Geometry check sheet. Reference: the model listing, model coordinates, mm. Face numbers are marked on the shaded views. A direction names the side the tool comes from. Coordinates: 2 decimals unless noted, no trailing zeros. Write each loop counter-clockwise with the first axis right and the second up, starting at its lowest first coordinate (ties: lowest second). Pieces come first, ordered by that corner, then holes. Notation, with made-up numbers: (-36.75, 60.5) -> (-30.75, 60.5) arc R29 cw to (-30.75, 89.5) -> close; hole circle Ø5 at (82, -12). An arc over 180 degrees is marked (long way). Answer as CSV lines item,"result".
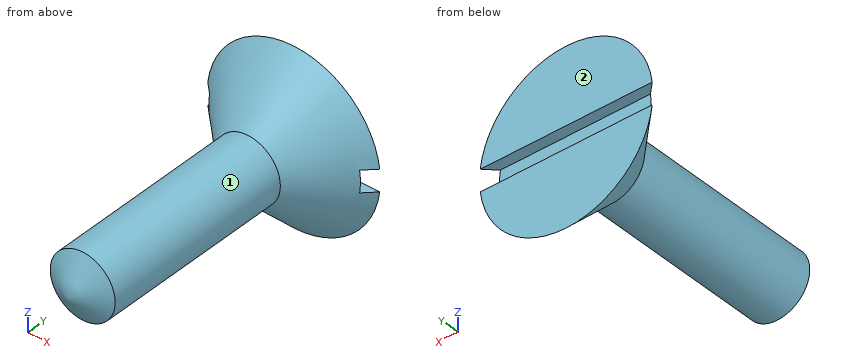
```python
from build123d import *

# Parameters (mm, degrees)
CUT_EXTRUDE1_DEPTH = 9


with BuildPart() as part:
    # Sketch1 → Revolve1 (revolve)
    with BuildSketch(Plane.XY):
        Polygon((0, 9), (0, -9), (0, -10.732050808), (3, -9), (3, 9), (8, 14), (0, 14), align=None)
    revolve(axis=Axis((0, 9, 0), (0, -1, 0)))

    # Sketch2 → Cut-Extrude1 (cut, symmetric)
    with BuildSketch(Plane(origin=(0, 0, 0), x_dir=(0, 0, -1), z_dir=(1, 0, 0))):
        Polygon((0, 14), (1, 14), (1, 13), (-1, 13), (-1, 14), align=None)
    extrude(amount=CUT_EXTRUDE1_DEPTH, both=True, mode=Mode.SUBTRACT)


solid = part.part
```
Item 1: Depth check by flat-ended pin: pin 1 Ø4 at (x, z) = (0.5, 4) entering from -Y; pin 2 Ø8 at (x, z) = (-3.5, 5.5) entering from -Y; pin 3 Ø0.6 at (x, z) = (1, 0) entering from +Y. Enter the tip coordinate at first touch or a pass-through.
Responses:
pin 1,"stops at y = -9.56"
pin 2,"stops at y = -9.28"
pin 3,"stops at y = 13"
Item 2: Thickness scan on probe 1 along Z at (x, y) = (3, 11.75); probe 2 along Y at (x, z) = (3, 2.75); probe 3 along Y at (x, z) = (2, 5.25). Record the ranges inside material, lowest first.
Responses:
probe 1,"z = -4.91 to 4.91"
probe 2,"y = 10.07 to 14"
probe 3,"y = 11.62 to 14"
Item 3: Cross-section at A-A, the plane y = 8.5. Record the cut outline in (x, z), plus the area to 3 significant figures.
Responses:
outline,"circle Ø6 at (0, 0)"
area,"28.3 mm2"
Item 4: Set-up check for the marked faces 1 and 2: record each of +Z, -Z, +X, -X, +Y, -Y from which the full face is reachable in a straight line by a thin tool's end or side.
Responses:
face 1,"-Y"
face 2,"+Z, -Z, +X, -X, +Y"
